from build123d import *

# Parameters (mm, degrees)
SKETCH_1_R          = 11.5
SKETCH_1_R_2        = 1
SKETCH_1_R_3        = 6
EXTRUDE_1_DEPTH     = 2.5
SKETCH_2_R          = 8.5
SKETCH_2_R_2        = 6
EXTRUDE_2_DEPTH     = 4
SKETCH_3_R          = 7.5
EXTRUDE_3_DEPTH     = 4
SKETCH_4_R          = 3.5
CUT_EXTRUDE_1_DEPTH = 4
SKETCH_6_R          = 0.25
CUT_EXTRUDE_2_DEPTH = 14
SKETCH_7_R          = 11.5
SKETCH_7_R_2        = 1
SKETCH_7_R_3        = 6
EXTRUDE_4_DEPTH     = 1
SKETCH_9_R          = 0.25
CUT_EXTRUDE_8_DEPTH = 12.2


with BuildPart() as part:
    # 草图1 → 凸台-拉伸1 (new body)
    with BuildSketch(Plane.XY):
        Circle(SKETCH_1_R)
        with Locations((9, 0)):
            Circle(SKETCH_1_R_2, mode=Mode.SUBTRACT)
        with Locations((2.781152949, -8.559508647)):
            Circle(SKETCH_1_R_2, mode=Mode.SUBTRACT)
        with Locations((-7.281152949, -5.290067271)):
            Circle(SKETCH_1_R_2, mode=Mode.SUBTRACT)
        with Locations((-7.281152949, 5.290067271)):
            Circle(SKETCH_1_R_2, mode=Mode.SUBTRACT)
        with Locations((2.781152949, 8.559508647)):
            Circle(SKETCH_1_R_2, mode=Mode.SUBTRACT)
        Circle(SKETCH_1_R_3, mode=Mode.SUBTRACT)
    extrude(amount=EXTRUDE_1_DEPTH)

    # 草图2 → 凸台-拉伸2 (add)
    with BuildSketch(Plane.XY.offset(2.5)):
        Circle(SKETCH_2_R)
        Circle(SKETCH_2_R_2, mode=Mode.SUBTRACT)
    extrude(amount=EXTRUDE_2_DEPTH)

    # 草图3 → 凸台-拉伸3 (add)
    with BuildSketch(Plane.XY.offset(6.5)):
        Circle(SKETCH_3_R)
    extrude(amount=EXTRUDE_3_DEPTH)

    # 草图4 → 切除-拉伸1 (cut)
    with BuildSketch(Plane.XY.offset(10.5)):
        Circle(SKETCH_4_R)
    extrude(amount=-CUT_EXTRUDE_1_DEPTH, mode=Mode.SUBTRACT)

    # 草图5 → 切除-旋转2 (revolve, cut)
    with BuildSketch(Plane(origin=(0, 0, 0), x_dir=(0, 0, -1), z_dir=(1, 0, 0))):
        Polygon((-7.5, 7.5), (-9.5, 7.5), (-8.75, 4.5), (-8.25, 4.5), (-6.5, 7.5), align=None)
    revolve(axis=Axis((0, 0, 10.5), (0, 0, -1)), mode=Mode.SUBTRACT)

    # 草图6 → 切除-拉伸2 (cut)
    with BuildSketch(Plane(origin=(0, 0, 0), x_dir=(1, 0, 0), z_dir=(0, 1, 0))):
        with Locations((0, -8.5)):
            Circle(SKETCH_6_R)
    extrude(amount=-CUT_EXTRUDE_2_DEPTH, mode=Mode.SUBTRACT)

    # 草图7 → 凸台-拉伸4 (add)
    with BuildSketch(Plane(origin=(0, 0, 0), x_dir=(-1, 0, 0), z_dir=(0, 0, -1))):
        Circle(SKETCH_7_R)
        with Locations((-2.781152949, -8.559508647)):
            Circle(SKETCH_7_R_2, mode=Mode.SUBTRACT)
        with Locations((7.281152949, -5.290067271)):
            Circle(SKETCH_7_R_2, mode=Mode.SUBTRACT)
        with Locations((7.281152949, 5.290067271)):
            Circle(SKETCH_7_R_2, mode=Mode.SUBTRACT)
        with Locations((-2.781152949, 8.559508647)):
            Circle(SKETCH_7_R_2, mode=Mode.SUBTRACT)
        with Locations((-9, 0)):
            Circle(SKETCH_7_R_2, mode=Mode.SUBTRACT)
        Circle(SKETCH_7_R_3, mode=Mode.SUBTRACT)
    extrude(amount=EXTRUDE_4_DEPTH)

    # 草图9 → 切除-拉伸8 (cut)
    with BuildSketch(Plane(origin=(0, 0, 0), x_dir=(0, 0, -1), z_dir=(1, 0, 0))):
        with Locations((-8.5, 0)):
            Circle(SKETCH_9_R)
    extrude(amount=-CUT_EXTRUDE_8_DEPTH, mode=Mode.SUBTRACT)


solid = part.part
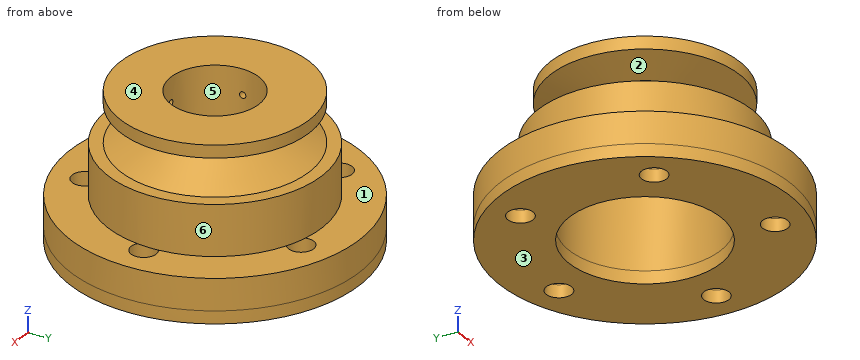
Model file for the job. Use its own axes, mm. Face numbers are marked on the shaded views. A direction names the side the tool comes from. Give positions to 0.01 mm unless a question says otherwise; leave off trailing zeros. Write each loop counter-clockwise with the first axis right and the second up, starting at its lowest first coordinate (ties: lowest second). Pieces come first, ordered by that corner, then holes. Notation, with made-up numbers: (-37.75, -32) -> (10.25, -32) arc R31 ccw to (10.25, -6) -> close; hole circle Ø11 at (48, 71.25). An arc over 180 degrees is marked (long way). Write item = value, one per line.
(1) Slice it at D-D, the plane x = 2.25. Give the number of separate pieces and of enclosed holes in the cut face, then the cut area to 3 significant figures.
Determined:
separate_pieces = 4
enclosed_holes = 0
area = 73.7 mm2
(2) Flat gauge pins, fed straight in: P1, Ø1.2, axis at x = -7.28, y = 5.29, coming from the -Z side; P2, Ø6, axis at x = 0.5, z = 6, coming from the +Y side; P3, Ø3, axis at x = -7, z = 5.5, coming from the -Y side. Where does each tip first touch, or does it go through?
Determined:
P1 = 2.5
P2 = 8.5
P3 = -6.48
(3) Tool access for the marked faces 1, 2 and 3: list every direction of +Z, -Z, +X, -X, +Y, -Y with a clear straight run to the whole face (end or side of a thin tool).
Determined:
face_1 = +Z
face_2 = none
face_3 = -Z, +X, -X, +Y, -Y
(4) Slice it at C-C, the plane z = 1.25. Give the cut face in (x, y).
Determined:
outline = circle Ø23 at (0, 0); hole circle Ø2 at (-7.28, -5.29); hole circle Ø2 at (-7.28, 5.29); hole circle Ø12 at (0, 0); hole circle Ø2 at (2.78, -8.56); hole circle Ø2 at (2.78, 8.56); hole circle Ø2 at (9, 0)
(5) Slice it at A-A, the plane x = 9. Give the cut face in (y, z), then the cut area to 3 significant figures.
Determined:
outline = (-7.16, -1) -> (-1, -1) -> (-1, 2.5) -> (-7.16, 2.5) -> close; (1, -1) -> (7.16, -1) -> (7.16, 2.5) -> (1, 2.5) -> close
area = 43.1 mm2
(6) Slice it at B-B, the plane z = 3.5. Give the cut face in (x, y).
Determined:
outline = circle Ø17 at (0, 0); hole circle Ø12 at (0, 0)
(7) Mould opens along Y. For the marked faces 4, 5 and 6 say: released by +Y, released by -Y, zero draft, split by the parting line, or undercut.
Determined:
face_4 = zero draft
face_5 = undercut
face_6 = split by the parting line
(8) Probe line 1 along X through (y, z) = (0, -0.7); line 2 along X through (y, z) = (-0.5, 0.25); line 3 along Z through (x, y) = (0, -4.15). List the from-to ranges inside material, lowest first.
Determined:
line_1 = -11.5 to -6, 6 to 8, 10 to 11.5
line_2 = -11.49 to -5.98, 5.98 to 8.13, 9.87 to 11.49
line_3 = 6.5 to 8.25, 8.75 to 10.5
